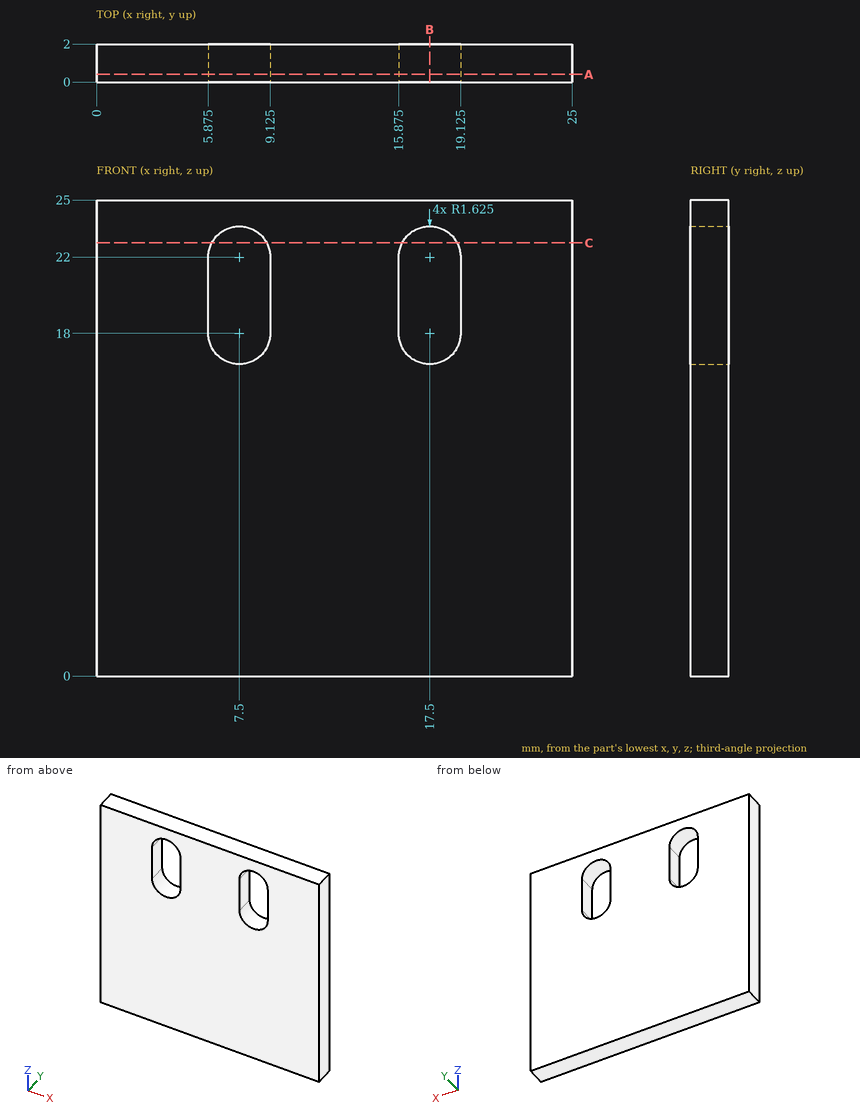
The figure shows three views and two pictorial views of one solid part (mm, origin at its lowest corner). Answer the questions. Coordinates: 2 decimals unless noted, no trailing zeros. Loops run counter-clockwise (first coordinate to the right, second up) from the corner with the lowest first, then second, coordinate; pieces in that order, holes last. Notation, with made-up numbers: (76, -37) -> (134, -37) arc R31 ccw to (134, -1) -> close; hole circle Ø3 at (45, -27). An arc over 180 degrees is marked (long way). Use one line per item in the form item = value. Start each with the question number.
Item 1: The part is cut by section A-A on y = 0.4. Determine the outline of the cut face in (x, z) (3 decimals).
Item 2: The part is cut by section C-C on z = 22.75. Determine the outline of the cut face in (x, y), then the cut area to 3 significant figures.
Item 3: Consider L1, parallel to X at y = 1.5, z = 20 (3 decimals); L2, parallel to Z at x = 17.5, y = 0.75 (3 decimals); L3, parallel to X at y = 1.8, z = 23.25. Determine where each line is inside the solid, lowest interval first. Write a range as [from, to].
Item 4: The part is cut by section B-B on x = 17.5. Determine the outline of the cut face in (y, z) (3 decimals).
Item 5: A flat-ended cylindrical pin translates along its axis: pin 1 Ø6 at (x, z) = (15, 6) entering from -Y. Find the tip coordinate at first contact, or state that the pin passes through.
Answer key:
q1.outline = (0, 0) -> (25, 0) -> (25, 25) -> (0, 25) -> close; hole (5.875, 18) arc R1.625 ccw to (9.125, 18) -> (9.125, 22) arc R1.625 ccw to (5.875, 22) -> close; hole (15.875, 18) arc R1.625 ccw to (19.125, 18) -> (19.125, 22) arc R1.625 ccw to (15.875, 22) -> close
q2.outline = (0, 0) -> (6.06, 0) -> (6.06, 2) -> (0, 2) -> close; (8.94, 0) -> (16.06, 0) -> (16.06, 2) -> (8.94, 2) -> close; (18.94, 0) -> (25, 0) -> (25, 2) -> (18.94, 2) -> close
q2.area = 38.5 mm2
q3.L1 = [0, 5.875], [9.125, 15.875], [19.125, 25]
q3.L2 = [0, 16.375], [23.625, 25]
q3.L3 = [0, 6.46], [8.54, 16.46], [18.54, 25]
q4.outline = (0, 0) -> (2, 0) -> (2, 16.375) -> (0, 16.375) -> close; (0, 23.625) -> (2, 23.625) -> (2, 25) -> (0, 25) -> close
q5.pin_1 = 0
